Build history of the part. All positions in model axes, mm. Face numbers are marked on the shaded views. Round coordinates to 2 decimals unless told otherwise and drop trailing zeros. Write each loop counter-clockwise with the first axis right and the second up, starting at its lowest first coordinate (ties: lowest second). Pieces come first, ordered by that corner, then holes. Notation, with made-up numbers: M -22,-21.75 L 12,-21.75 A13 cw 12,-3.75 Z; hole C -2.5,80 d2. An arc over 180 degrees is marked long. One line per item, written item: value. Start each with the question number.
```python
from build123d import *

# Parameters (mm, degrees)
BOSS_EXTRUDE1_DEPTH = 35
CUT_EXTRUDE2_DEPTH  = 36
BOSS_EXTRUDE2_DEPTH = 0.4
FILLET1_R           = 8


with BuildPart() as part:
    # Sketch1 → Boss-Extrude1 (new body)
    with BuildSketch(Plane(origin=(0, 0, 0), x_dir=(1, 0, 0), z_dir=(0, 1, 0))):
        with BuildLine():
            ThreePointArc((1.451818925, -34.068556857), (1.641248992, -34.346908706), (1.964225605, -34.442038138))
            ThreePointArc((1.964225605, -34.442038138), (26.591847487, -21.978073076), (34.198225299, 4.555174015))
            ThreePointArc((34.198225299, 4.555174015), (23.590291339, 25.176355888), (2.324135821, 34.423627607))
            ThreePointArc((2.324135821, 34.423627607), (1.751838249, 34.289058819), (1.354061739, 33.856153382))
            ThreePointArc((1.354061739, 33.856153382), (0, 33.001534515), (-1.354061739, 33.856153382))
            ThreePointArc((-1.354061739, 33.856153382), (-1.751838249, 34.289058819), (-2.324135821, 34.423627607))
            ThreePointArc((-2.324135821, 34.423627607), (-23.590291339, 25.176355888), (-34.198225299, 4.555174015))
            ThreePointArc((-34.198225299, 4.555174015), (-26.591847487, -21.978073076), (-1.964225605, -34.442038138))
            ThreePointArc((-1.964225605, -34.442038138), (-1.641248992, -34.346908706), (-1.451818925, -34.068556857))
            ThreePointArc((-1.451818925, -34.068556857), (0, -32.945679925), (1.451818925, -34.068556857))
        make_face()
        with BuildLine():
            Line((-2.417, 3.787737139), (0, 3.787737139))
            Line((0, 3.787737139), (2.417, 3.787737139))
            ThreePointArc((2.417, 3.787737139), (0, -4.489512172), (-2.417, 3.787737139))
        make_face(mode=Mode.SUBTRACT)
    extrude(amount=BOSS_EXTRUDE1_DEPTH)

    # Sketch2 → Cut-Extrude2 (cut, through all)
    with BuildSketch(Plane(origin=(0, 0, 0), x_dir=(1, 0, 0), z_dir=(0, 1, 0))):
        with BuildLine():
            ThreePointArc((-24.771875163, 3.369599515), (-23.997809329, -7.007506505), (-19.066036357, -16.170536714))
            ThreePointArc((-19.066036357, -16.170536714), (-12.361903527, -15.700472812), (-11.245933621, -22.327762472))
            ThreePointArc((-11.245933621, -22.327762472), (-0.884127319, -24.984361486), (9.639544373, -23.066841662))
            ThreePointArc((9.639544373, -23.066841662), (10.917339043, -16.055130989), (17.907795118, -17.44450842))
            ThreePointArc((17.907795118, -17.44450842), (23.625967237, -8.17396306), (24.859344713, 2.64820325))
            ThreePointArc((24.859344713, 2.64820325), (18.515062391, 5.879189473), (21.833190005, 12.178333803))
            ThreePointArc((21.833190005, 12.178333803), (14.752111216, 20.18353821), (4.974937186, 24.5))
            ThreePointArc((4.974937186, 24.5), (0, 20), (-4.974937186, 24.5))
            ThreePointArc((-4.974937186, 24.5), (-14.514359509, 20.355180374), (-21.541517866, 12.687119769))
            ThreePointArc((-21.541517866, 12.687119769), (-19.215771141, 6.662052225), (-24.771875163, 3.369599515))
        make_face()
    extrude(amount=CUT_EXTRUDE2_DEPTH, mode=Mode.SUBTRACT)

    # Sketch2<2> → Boss-Extrude2 (add)
    with BuildSketch(Plane(origin=(0, 0, 0), x_dir=(1, 0, 0), z_dir=(0, 1, 0))):
        with BuildLine():
            ThreePointArc((-24.771875163, 3.369599515), (-23.997809329, -7.007506505), (-19.066036357, -16.170536714))
            ThreePointArc((-19.066036357, -16.170536714), (-12.361903527, -15.700472812), (-11.245933621, -22.327762472))
            ThreePointArc((-11.245933621, -22.327762472), (-0.884127319, -24.984361486), (9.639544373, -23.066841662))
            ThreePointArc((9.639544373, -23.066841662), (10.917339043, -16.055130989), (17.907795118, -17.44450842))
            ThreePointArc((17.907795118, -17.44450842), (23.625967237, -8.17396306), (24.859344713, 2.64820325))
            ThreePointArc((24.859344713, 2.64820325), (18.515062391, 5.879189473), (21.833190005, 12.178333803))
            ThreePointArc((21.833190005, 12.178333803), (14.752111216, 20.18353821), (4.974937186, 24.5))
            ThreePointArc((4.974937186, 24.5), (0, 20), (-4.974937186, 24.5))
            ThreePointArc((-4.974937186, 24.5), (-14.514359509, 20.355180374), (-21.541517866, 12.687119769))
            ThreePointArc((-21.541517866, 12.687119769), (-19.215771141, 6.662052225), (-24.771875163, 3.369599515))
        make_face()
    extrude(amount=BOSS_EXTRUDE2_DEPTH)

    # Fillet1
    fillet1_edges = [part.edges().sort_by_distance(p)[0] for p in [
        (14.752111216, 0.4, -20.18353821),
        (0, 0.4, -20),
        (-14.514359509, 0.4, -20.355180374),
        (-19.215771141, 0.4, -6.662052225),
        (-23.997809329, 0.4, 7.007506505),
        (-12.361903527, 0.4, 15.700472812),
        (-0.884127319, 0.4, 24.984361486),
        (10.917339043, 0.4, 16.055130989),
        (23.625967237, 0.4, 8.17396306),
        (18.515062391, 0.4, -5.879189473),
    ]]
    fillet(fillet1_edges, radius=FILLET1_R)


solid = part.part
```
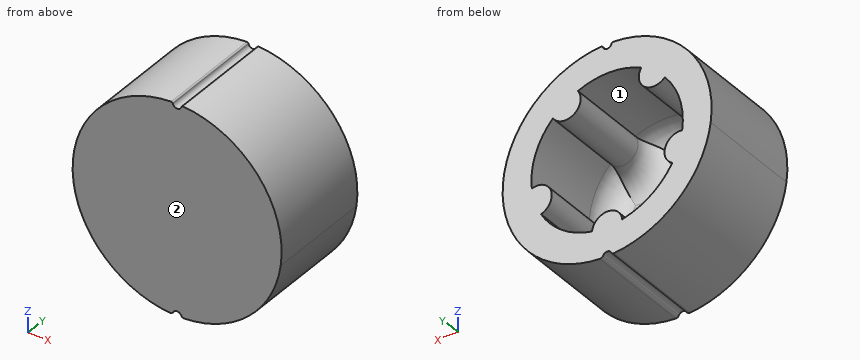
Item 1: Cut at C-C, the plane x = 29.5. Write the cut outline in (y, z), plus the area to 3 significant figures.
Item 2: Drill centre lines: line 1 (Z direction, x = 9.5, y = 20.5); line 2 (Z direction, x = 21, y = 28); line 3 (X direction, y = 27.5, z = 7.5). Where is each one in solid material? Low to high.
Item 3: Cut at B-B, the plane z = -29. Write the cut outline in (x, y), plus the area to 3 significant figures.
Item 4: Drop flat-ended pins along their axis: pin 1 (6 mm diameter, centred on y = 21, z = -9, fed in from -X); pin 2 (12 mm diameter, centred on x = -9.5, y = 18, fed in from +Z); pin 3 (3 mm diameter, centred on x = 7.5, z = -19.5, fed in from +Y). Give the stop position or say it passes through.
Item 5: Two-plate mould, pull along Z, no slides. Class the marked faces 1 and 2: pulls with the +Z half, pulls with the -Z half, needs draft (parallel to the pull), parting line crosses it, or undercut.
Computed values:
1. outline: M 0,-17.89 L 35,-17.89 L 35,17.89 L 0,17.89 Z
1. area: 1,250 mm2
2. line 1: z = -33.17 to -23.12, 17.52 to 22.86, 23.12 to 33.16
2. line 2: z = -27.37 to -13.56, -11.84 to -2.94, 13.56 to 27.37
2. line 3: x = -33.67 to -23.85, 23.85 to 33.67
3. outline: M -18.69,0 L 18.69,0 L 18.69,35 L -18.69,35 Z
3. area: 1,310 mm2
4. pin 1: stops at x = -33.97
4. pin 2: stops at z = 34.32
4. pin 3: stops at y = 2.49
5. face 1: undercut
5. face 2: needs draft
